Read the model definition and answer for the solid it produces. Units are mm, in the model's axes. A direction names the side the tool comes from. Round coordinates to 2 decimals unless told otherwise and drop trailing zeros. Loops run counter-clockwise (first coordinate to the right, second up) from the corner with the lowest first, then second, coordinate; pieces in that order, holes last. Notation, with made-up numbers: (14.25, 65) - (69.25, 65) arc R21 ccw to (69.25, 85) - close; hole circle Ø4 at (19.5, -34). An arc over 180 degrees is marked (long way). Use CSV: the item, a comma, the result in double quotes. Start each with the question number.
1. Given pin 1 Ø5 at (x, z) = (-3, 4.5) entering from +Y; pin 2 Ø2 at (x, z) = (40.5, 4) entering from +Y; pin 3 Ø1 at (y, z) = (-84, 3.5) entering from -X, each flat-ended and moving along its own axis, determine where each tip first touches the part or whether it passes through.
2. Find section A-A (y = -7.5). Give the vertices of the cut face in (x, z).
3. A tool of negligible diameter and unlimited length cuts with its end or side. For faces 1 (the flat face through (1, -101, 2.311)), 2 (the flat face through (-72.585, -1.422, 6.261)), from which of +Z, -Z, +X, -X, +Y, -Y can it reach the whole face along a straight path? Write none if from no direction.
4. Consider line 1 along Y through (x, z) = (0, 1.4); line 2 along Y through (x, z) = (0, 0.5); line 3 along X through (y, z) = (-14, 1.75). Determine where each line is inside the solid, lowest interval first.
5. Find section B-B (x = -62). Give the vertices of the cut face in (y, z).
from build123d import *

# Parameters (mm, degrees)
F0_W     = 152.4
F0_H     = 203.2
F1_DEPTH = 12.7
F1_TAPER = 30
F2_W     = 6.35
F2_H     = 1.5690360503
F3_DEPTH = 2.3114
F4_R     = 1.905
F5_DEPTH = 25.4


with BuildPart() as f1:
    # F0 (on Top) → F1 (new body)
    with BuildSketch(Plane.XY):
        Rectangle(F0_W, F0_H)
    extrude(amount=F1_DEPTH, taper=F1_TAPER)

    # F2 (on face) → F3 (join)
    with BuildSketch(Plane(origin=(0, 0, 0), x_dir=(1, 0, 0), z_dir=(0, 0, -1))):
        with BuildLine():
            Line((-3.175, 101.6), (3.175, 101.6))
            Line((3.175, 101.6), (3.175, 103.2059639497))
            ThreePointArc((3.175, 103.2059639497), (1.125e-07, 106.3809639692), (-3.175, 103.2059641746))
            Line((-3.175, 103.2059641746), (-3.175, 101.6))
        make_face()
        with Locations((0, 100.8154819748)):
            Rectangle(F2_W, F2_H)
    extrude(amount=-F3_DEPTH)

    # F4 (on face) → F5 (cut)
    with BuildSketch(Plane.XY.offset(2.3114)):
        with Locations((0, -103.2059639692)):
            Circle(F4_R)
    extrude(amount=-F5_DEPTH, mode=Mode.SUBTRACT)


solid = f1.part
Filled sheet:
1,pin 1,"stops at y = 100.45"
1,pin 2,"stops at y = 99.87"
1,pin 3,"stops at x = -74.47"
2,outline,"(-76.2, 0) - (76.2, 0) - (68.87, 12.7) - (-68.87, 12.7) - close"
3,face 1,"+Z, +X, -X, -Y"
3,face 2,"+Z, -X, +Y, -Y"
4,line 1,"y = -106.38 to -105.11, -101.3 to 100.79"
4,line 2,"y = -106.38 to -105.11, -101.3 to 101.31"
4,line 3,"x = -75.19 to 75.19"
5,outline,"(-101.6, 0) - (101.6, 0) - (94.27, 12.7) - (-94.27, 12.7) - close"
